The listing builds one solid part. Answer for the finished solid, in the listing's coordinates (mm). A direction names the side the tool comes from. Round coordinates to 2 decimals unless told otherwise and drop trailing zeros. Loops run counter-clockwise (first coordinate to the right, second up) from the corner with the lowest first, then second, coordinate; pieces in that order, holes last. Notation, with made-up numbers: M 45.5,-34 L 85.5,-34 A23 ccw 85.5,-8 Z; hole C 65,-6.75 d11. An arc over 180 degrees is marked long. Put each result on its own line as item: value. Start each with the question number.
(1) Straight lines are drawn through the part: line 1 (Z direction, x = 13, y = 1); line 2 (Z direction, x = -11.5, y = -9.5); line 3 (Z direction, x = 15.5, y = -9). For each, find the intervals that lie inside material, in ascending order.
(2) Section D-D, the plane x = 9 is taken. Determine the outline of the cut face in (y, z).
(3) Section C-C, the plane y = 10.5 is taken. Determine the outline of the cut face in (x, z).
(4) Determine the mould class of faces 5 (the face through (-16.374, 14.901, 5.821)), 6 (the face through (15, -20.799, 1)), 7 (the face through (-1, -29.117, 8)) for opening direction X: released by +X, released by -X, zero draft, split by the parting line, or undercut.
(5) Flat-ended cylindrical pins translate along their axes: P1, Ø3, axis at x = -9, y = -20, coming from the -Z side; P2, Ø2.5, axis at x = -12, y = 13.5, coming from the -Z side; P3, Ø1.3, axis at y = 14, z = -2.5, coming from the -X side. Find the tip coordinate at first contact, or state that the pin passes through.
(6) Section B-B, the plane x = -2 is taken. Determine the outline of the cut face in (y, z), then the cut area to 3 significant figures.
(7) Which of the six approach directions +Z, -Z, +X, -X, +Y, -Y give full straight-line access (tool end or side, diameter ignored) to faces 1 (the face through (13.866, 12.955, -2.49)), 2 (the face through (-10, 13, -2.1)), 3 (the face through (10, 13, -2.1)), 4 (the face through (-7, 13.7, -2.3))?
(8) Section A-A, the plane z = 4 is taken. Determine the outline of the cut face in (x, y), then the cut area to 3 significant figures.
```python
from build123d import *

# Parameters (mm, degrees)
EXTRUDE_1_DEPTH      = 15
EXTRUDE_2_DEPTH      = 2
SKETCH_3_W           = 2
SKETCH_3_H           = 30
EXTRUDE_3_DEPTH      = 2
SKETCH_4_W           = 2
SKETCH_4_H           = 30
EXTRUDE_4_DEPTH      = 2
EXTRUDE_START        = 7
EXTRUDE_5_DEPTH      = 5.5
EXTRUDE_6_DEPTH      = 7.3
EXTRUDE_6_DEPTH_BACK = 16
EXTRUDE_7_DEPTH      = 23.3
EXTRUDE_9_DEPTH      = 5.05
CUT_EXTRUDE_3_DEPTH  = 8.15


with BuildPart() as part:
    # Sketch 1 → Extrude 1 (new body)
    with BuildSketch(Plane.XY):
        Polygon((-18.227330455, -27.306853771), (-16.416835991, -29.117348235), (15.781834721, -29.117348235), (18.100330201, -26.798852755), (18.100330201, 12.794403278), (14.191406072, 16.703327407), (-14.572406834, 16.703327407), (-18.227330455, 13.048403786), align=None)
        with BuildLine():
            ThreePointArc((-15.190500381, -26.798852755), (-15.897607162, -26.505959536), (-16.190500381, -25.798852755))
            Line((-16.190500381, -25.798852755), (-16.190500381, 11.201147245))
            ThreePointArc((-16.190500381, 11.201147245), (-15.897607162, 11.908254026), (-15.190500381, 12.201147245))
            Line((-15.190500381, 12.201147245), (14.809499619, 12.201147245))
            ThreePointArc((14.809499619, 12.201147245), (15.5166064, 11.908254026), (15.809499619, 11.201147245))
            Line((15.809499619, 11.201147245), (15.809499619, -25.798852755))
            ThreePointArc((15.809499619, -25.798852755), (15.5166064, -26.505959536), (14.809499619, -26.798852755))
            Line((14.809499619, -26.798852755), (-15.190500381, -26.798852755))
        make_face(mode=Mode.SUBTRACT)
    extrude(amount=EXTRUDE_1_DEPTH)

    # Sketch 2 → Extrude 2 (add)
    with BuildSketch(Plane.XY.offset(15)):
        Polygon((14.191406072, 16.703327407), (-14.572406834, 16.703327407), (-18.227330455, 13.048403786), (-18.227330455, -27.306853771), (-16.416835991, -29.117348235), (-0.317500635, -29.117348235), (15.781834721, -29.117348235), (18.100330201, -26.798852755), (18.100330201, 12.794403278), align=None)
    extrude(amount=EXTRUDE_2_DEPTH)

    # Sketch 3 → Extrude 3 (add)
    with BuildSketch(Plane(origin=(-16.190500381, 0, 0), x_dir=(0, 0, -1), z_dir=(1, 0, 0))):
        with Locations((-1, -5.798852755)):
            Rectangle(SKETCH_3_W, SKETCH_3_H)
    extrude(amount=EXTRUDE_3_DEPTH)

    # Sketch 4 → Extrude 4 (add)
    with BuildSketch(Plane.ZY.offset(-15.809499619)):
        with Locations((1, -5.798852755)):
            Rectangle(SKETCH_4_W, SKETCH_4_H)
    extrude(amount=EXTRUDE_4_DEPTH)

    # Sketch 5 → Extrude 5 (add)
    with BuildSketch(Plane(origin=(0, 0, 0), x_dir=(0, 0, -1), z_dir=(1, 0, 0)).offset(EXTRUDE_START)):
        Polygon((0, 14.003327407), (0, 15.353327407), (3.1000508, 15.353327407), (3.1000508, 12.703327407), (2.1000508, 12.703327407), (2.1000508, 13.703327407), (2.1000508, 14.003327407), align=None)
    extrude_5 = extrude(amount=EXTRUDE_5_DEPTH)

    # Mirror 1: Extrude 5 across plane
    add(extrude_5.mirror(Plane(origin=(0, 0, 0), x_dir=(0, 0, 1), z_dir=(1, 0, 0))))

    # Sketch 7 → Extrude 6 (add, two sides: drawn at the far end of the back side and taken through both)
    with BuildSketch(Plane(origin=(0, 0, 0), x_dir=(1, 0, 0), z_dir=(0, 1, 0)).offset(-EXTRUDE_6_DEPTH_BACK)):
        Polygon((-18.227330455, 3.1), (-18.227330455, 0), (-15.477330455, 0), (-15.477330455, 2.1000508), (-15.227330455, 2.1000508), (-11.227330455, 2.1000508), (-11.227330455, 3.1), (-16.227330455, 3.1), (-16.227330455, 4.1), (-11.227330455, 4.1), (-11.227330455, 5.1), (-18.227330455, 5.1), (-18.227330455, 4.1), align=None)
    extrude(amount=EXTRUDE_6_DEPTH + EXTRUDE_6_DEPTH_BACK)

    # Sketch 10 → Extrude 7 (add)
    with BuildSketch(Plane.XZ.offset(16)):
        Polygon((16.227721063, -3.100000069), (11.227330455, -3.100000069), (11.227330455, -2.048141563), (15.600330201, -2.048141563), (15.600330201, -1.6000508), (15.600330201, 0), (16.226569186, 0.001858295), (18.100330201, 0), (18.100330201, -5.1), (11.227330455, -5.1), (11.227330455, -4.1), (16.228092414, -4.1), align=None)
    extrude(amount=-EXTRUDE_7_DEPTH)

    # Sketch 11 → Extrude 9 (add)
    with BuildSketch(Plane(origin=(0, 0, 0), x_dir=(-1, 0, 0), z_dir=(0, 0, -1))):
        Polygon((-15.220330201, 7.12413323), (-18.100330201, 7.12413323), (-18.100330201, 12.794403278), (-14.191406072, 16.703327407), (14.572406834, 16.703327407), (18.227330455, 13.048403786), (18.227330455, 7.12413323), (15.347330455, 7.12413323), (15.347330455, 11.855468727), (13.414618961, 13.78818022), (12.930706389, 14.272092792), (-12.549705627, 14.272092792), (-15.220330201, 11.601468219), align=None)
    extrude(amount=EXTRUDE_9_DEPTH)

    # Sketch 14 → Cut-Extrude 3 (cut)
    # profile 1 of 4: a face of its own
    with BuildSketch(Plane(origin=(0, 16.703327407, 0), x_dir=(1, 0, 0), z_dir=(0, 1, 0))):
        with BuildLine():
            ThreePointArc((3.273301705, 0.219606282), (4.147281949, -0.142408188), (4.509296419, -1.016388431))
            Line((4.509296419, -1.016388431), (4.509296419, -2.139582087))
            ThreePointArc((4.509296419, -2.139582087), (4.147281949, -3.01356233), (3.273301705, -3.3755768))
            Line((3.273301705, -3.3755768), (-3.222501604, -3.3755768))
            ThreePointArc((-3.222501604, -3.3755768), (-4.096481847, -3.01356233), (-4.458496317, -2.139582087))
            Line((-4.458496317, -2.139582087), (-4.458496317, -1.016388431))
            ThreePointArc((-4.458496317, -1.016388431), (-4.096481847, -0.142408188), (-3.222501604, 0.219606282))
            Line((-3.222501604, 0.219606282), (3.273301705, 0.219606282))
        make_face()
        with BuildLine():
            Line((3.273301705, -0.080393718), (-3.222501604, -0.080393718))
            ThreePointArc((-3.222501604, -0.080393718), (-3.884349813, -0.354540222), (-4.158496317, -1.016388431))
            Line((-4.158496317, -1.016388431), (-4.158496317, -2.139582087))
            ThreePointArc((-4.158496317, -2.139582087), (-3.884349813, -2.801430296), (-3.222501604, -3.0755768))
            Line((-3.222501604, -3.0755768), (3.273301705, -3.0755768))
            ThreePointArc((3.273301705, -3.0755768), (3.935149914, -2.801430296), (4.209296419, -2.139582087))
            Line((4.209296419, -2.139582087), (4.209296419, -1.016388431))
            ThreePointArc((4.209296419, -1.016388431), (3.935149914, -0.354540222), (3.273301705, -0.080393718))
        make_face(mode=Mode.SUBTRACT)
    # profile 2 of 4: a face of its own
    with BuildSketch(Plane(origin=(0, 16.703327407, 0), x_dir=(1, 0, 0), z_dir=(0, 1, 0))):
        with BuildLine():
            ThreePointArc((3.273301705, -0.080393718), (3.935149914, -0.354540222), (4.209296419, -1.016388431))
            Line((4.209296419, -1.016388431), (4.209296419, -2.139582087))
            ThreePointArc((4.209296419, -2.139582087), (3.935149914, -2.801430296), (3.273301705, -3.0755768))
            Line((3.273301705, -3.0755768), (-3.222501604, -3.0755768))
            ThreePointArc((-3.222501604, -3.0755768), (-3.884349813, -2.801430296), (-4.158496317, -2.139582087))
            Line((-4.158496317, -2.139582087), (-4.158496317, -1.016388431))
            ThreePointArc((-4.158496317, -1.016388431), (-3.884349813, -0.354540222), (-3.222501604, -0.080393718))
            Line((-3.222501604, -0.080393718), (3.273301705, -0.080393718))
        make_face()
    # profile 3 of 4: a face of its own
    with BuildSketch(Plane(origin=(0, 16.703327407, 0), x_dir=(1, 0, 0), z_dir=(0, 1, 0))):
        with BuildLine():
            Line((4.509296419, 0.219606282), (3.273301705, 0.219606282))
            ThreePointArc((3.273301705, 0.219606282), (4.147281949, -0.142408188), (4.509296419, -1.016388431))
            Line((4.509296419, -1.016388431), (4.509296419, 0.219606282))
        make_face()
    # profile 4 of 4: a face of its own
    with BuildSketch(Plane(origin=(0, 16.703327407, 0), x_dir=(1, 0, 0), z_dir=(0, 1, 0))):
        with BuildLine():
            Line((-4.458496317, -1.016388431), (-4.470508001, 0.219606282))
            Line((-4.470508001, 0.219606282), (-3.222501604, 0.219606282))
            ThreePointArc((-3.222501604, 0.219606282), (-4.096481847, -0.142408188), (-4.458496317, -1.016388431))
        make_face()
    extrude(amount=-CUT_EXTRUDE_3_DEPTH, mode=Mode.SUBTRACT)


solid = part.part
```
Recorded:
1. line 1: z = -5.1 to -4.1, -3.1 to -2.05, 15 to 17
1. line 2: z = -5.1 to -4.1, -3.1 to -2.1, 15 to 17
1. line 3: z = -5.1 to -4.1, -3.1 to -2.05, 0 to 2, 15 to 17
2. outline: M -29.12,0 L -26.8,0 L -26.8,15 L 12.2,15 L 12.2,0 L 14,0 L 14,-2.1 L 12.7,-2.1 L 12.7,-3.1 L 14.27,-3.1 L 14.27,-5.05 L 16.7,-5.05 L 16.7,17 L -29.12,17 Z
3. outline: M -18.23,-5.05 L -15.35,-5.05 L -15.35,0 L -16.19,0 L -16.19,15 L 15.81,15 L 15.81,0 L 15.22,0 L 15.22,-5.05 L 18.1,-5.05 L 18.1,17 L -18.23,17 Z
4. face 5: released by -X
4. face 6: undercut
4. face 7: zero draft
5. P1: stops at z = 15
5. P2: stops at z = -5.05
5. P3: stops at x = -17.93
6. outline: M -29.12,0 L -26.8,0 L -26.8,15 L 12.2,15 L 12.2,3.38 L 16.7,3.38 L 16.7,17 L -29.12,17 Z; M 14.27,-5.05 L 16.7,-5.05 L 16.7,-0.22 L 14.27,-0.22 Z
6. area: 190 mm²
7. face 1: -Z
7. face 2: -Y
7. face 3: none
7. face 4: -Z, -Y
8. outline: M -18.23,-27.31 L -16.42,-29.12 L 15.78,-29.12 L 18.1,-26.8 L 18.1,12.79 L 14.19,16.7 L -14.57,16.7 L -18.23,13.05 Z; hole M -16.19,-25.8 A1 ccw -15.19,-26.8 L 14.81,-26.8 A1 ccw 15.81,-25.8 L 15.81,11.2 A1 ccw 14.81,12.2 L -15.19,12.2 A1 ccw -16.19,11.2 Z
8. area: 399 mm²
